Model file for the job. Use its own axes, mm. Coordinates: 2 decimals unless noted, no trailing zeros. Order: outer loops, then holes, each group sorted by start corner. A loop starts at its lowest first (then second) coordinate and runs counter-clockwise, first axis right, second up.
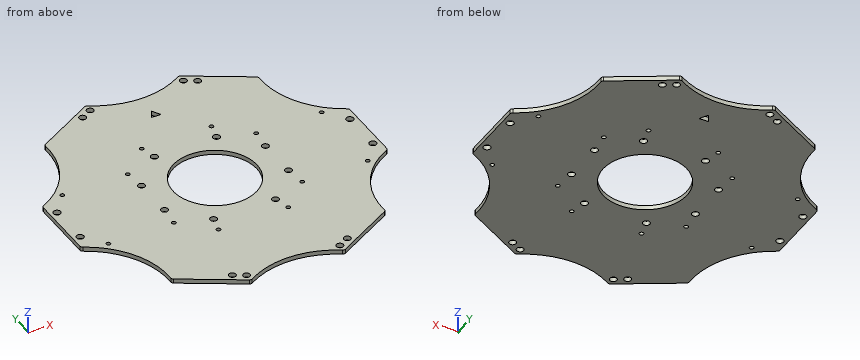
from build123d import *

# Parameters (mm, degrees)
SKETCH1_R           = 2.5
SKETCH1_R_2         = 2.6
SKETCH1_R_3         = 1.5
SKETCH1_R_4         = 30
BOSS_EXTRUDE1_DEPTH = 3.175
FILLET1_R           = 2


with BuildPart() as part:
    # Sketch1 → Boss-Extrude1 (new body)
    with BuildSketch(Plane.XY):
        with BuildLine():
            Line((-120, -25), (-120, 25))
            ThreePointArc((-120, 25), (-94.559451613, 48.820422151), (-86.650635095, 82.762794416))
            Line((-86.650635095, 82.762794416), (-43.349364905, 107.762794416))
            ThreePointArc((-43.349364905, 107.762794416), (-10, 97.640844302), (23.349364905, 107.762794416))
            Line((23.349364905, 107.762794416), (66.650635095, 82.762794416))
            ThreePointArc((66.650635095, 82.762794416), (74.559451613, 48.820422151), (100, 25))
            Line((100, 25), (100, -25))
            ThreePointArc((100, -25), (74.559451613, -48.820422151), (66.650635095, -82.762794416))
            Line((66.650635095, -82.762794416), (23.349364905, -107.762794416))
            ThreePointArc((23.349364905, -107.762794416), (-10, -97.640844302), (-43.349364905, -107.762794416))
            Line((-43.349364905, -107.762794416), (-86.650635095, -82.762794416))
            ThreePointArc((-86.650635095, -82.762794416), (-94.559451613, -48.820422151), (-120, -25))
        make_face()
        with Locations((12.227985364, -38.5)):
            Circle(SKETCH1_R, mode=Mode.SUBTRACT)
        with Locations((-54.455970728, 15)):
            Circle(SKETCH1_R, mode=Mode.SUBTRACT)
        with Locations((12.227985364, 38.5)):
            Circle(SKETCH1_R_2, mode=Mode.SUBTRACT)
        with Locations((-32.227985364, 38.5)):
            Circle(SKETCH1_R_2, mode=Mode.SUBTRACT)
        with Locations((-54.455970728, -15)):
            Circle(SKETCH1_R, mode=Mode.SUBTRACT)
        with Locations((-32.227985364, -38.5)):
            Circle(SKETCH1_R, mode=Mode.SUBTRACT)
        with Locations((95, 15)):
            Circle(SKETCH1_R_2, mode=Mode.SUBTRACT)
        with Locations((95, -15)):
            Circle(SKETCH1_R_2, mode=Mode.SUBTRACT)
        with Locations((-115, -15)):
            Circle(SKETCH1_R_2, mode=Mode.SUBTRACT)
        with Locations((-115, 15)):
            Circle(SKETCH1_R_2, mode=Mode.SUBTRACT)
        with Locations((31.241669751, -97.432667397)):
            Circle(SKETCH1_R, mode=Mode.SUBTRACT)
        with Locations((23.447441117, -101.932667397)):
            Circle(SKETCH1_R, mode=Mode.SUBTRACT)
        with Locations((-43.447441117, -101.932667397)):
            Circle(SKETCH1_R, mode=Mode.SUBTRACT)
        with Locations((-51.241669751, -97.432667397)):
            Circle(SKETCH1_R, mode=Mode.SUBTRACT)
        with Locations((-51.241669751, 97.432667397)):
            Circle(SKETCH1_R, mode=Mode.SUBTRACT)
        with Locations((-43.447441117, 101.932667397)):
            Circle(SKETCH1_R, mode=Mode.SUBTRACT)
        with Locations((23.447441117, 101.932667397)):
            Circle(SKETCH1_R, mode=Mode.SUBTRACT)
        with Locations((31.241669751, 97.432667397)):
            Circle(SKETCH1_R, mode=Mode.SUBTRACT)
        with Locations((34.455970728, -15)):
            Circle(SKETCH1_R, mode=Mode.SUBTRACT)
        with Locations((34.455970728, 15)):
            Circle(SKETCH1_R, mode=Mode.SUBTRACT)
        with Locations((-103, 30)):
            Circle(SKETCH1_R_3, mode=Mode.SUBTRACT)
        with Locations((-56, 30)):
            Circle(SKETCH1_R_3, mode=Mode.SUBTRACT)
        with Locations((-56, -30)):
            Circle(SKETCH1_R_3, mode=Mode.SUBTRACT)
        with Locations((-103, -30)):
            Circle(SKETCH1_R_3, mode=Mode.SUBTRACT)
        with Locations((36, 30)):
            Circle(SKETCH1_R_3, mode=Mode.SUBTRACT)
        with Locations((36, -30)):
            Circle(SKETCH1_R_3, mode=Mode.SUBTRACT)
        with Locations((83, 30)):
            Circle(SKETCH1_R_3, mode=Mode.SUBTRACT)
        with Locations((83, -30)):
            Circle(SKETCH1_R_3, mode=Mode.SUBTRACT)
        with Locations((-35, 50)):
            Circle(SKETCH1_R_3, mode=Mode.SUBTRACT)
        with Locations((15, 50)):
            Circle(SKETCH1_R_3, mode=Mode.SUBTRACT)
        with Locations((15, -50)):
            Circle(SKETCH1_R_3, mode=Mode.SUBTRACT)
        with Locations((-35, -50)):
            Circle(SKETCH1_R_3, mode=Mode.SUBTRACT)
        with Locations((-10, 0)):
            Circle(SKETCH1_R_4, mode=Mode.SUBTRACT)
        Polygon((-10, 82.640844302), (-13.464101615, 76.640844302), (-6.535898385, 76.640844302), align=None, mode=Mode.SUBTRACT)
    extrude(amount=BOSS_EXTRUDE1_DEPTH)

    # Fillet1
    fillet1_edges = [part.edges().sort_by_distance(p)[0] for p in [
        (-120, -25, 1.5875),
        (-120, 25, 1.5875),
        (-86.650635095, 82.762794416, 1.5875),
        (-43.349364905, 107.762794416, 1.5875),
        (23.349364905, 107.762794416, 1.5875),
        (66.650635095, 82.762794416, 1.5875),
        (100, 25, 1.5875),
        (100, -25, 1.5875),
        (66.650635095, -82.762794416, 1.5875),
        (23.349364905, -107.762794416, 1.5875),
        (-43.349364905, -107.762794416, 1.5875),
        (-86.650635095, -82.762794416, 1.5875),
    ]]
    fillet(fillet1_edges, radius=FILLET1_R)


solid = part.part
Q1. Probe line 1 (Y direction, x = 22, z = 1.6); line 2 (Y direction, x = 36, z = 0.9); line 3 (X direction, y = 30.5, z = 2.4). List the from-to ranges inside material, lowest first.
Established:
line 1: y = -106.89 to -103.97, -99.89 to 99.89, 103.97 to 106.89
line 2: y = -100.46 to -31.5, -28.5 to -16.97, -13.03 to 13.03, 16.97 to 28.5, 31.5 to 100.46
line 3: x = -110.95 to -104.41, -101.59 to -57.41, -54.59 to 34.59, 37.41 to 81.59, 84.41 to 90.95
Q2. Cut at A-A, the plane x = 95. List the corners of the cut face in (y, z) (3 decimals), plus the area to 3 significant figures.
Established:
outline: (-27.767, 0) - (-17.6, 0) - (-17.6, 3.175) - (-27.767, 3.175) - close; (-12.4, 0) - (12.4, 0) - (12.4, 3.175) - (-12.4, 3.175) - close; (17.6, 0) - (27.767, 0) - (27.767, 3.175) - (17.6, 3.175) - close
area: 143 mm2
Q3. Cut at B-B, the plane y = 38.5. List the corners of the cut face in (x, z) (3 decimals).
Established:
outline: (-102.088, 0) - (-34.828, 0) - (-34.828, 3.175) - (-102.088, 3.175) - close; (-29.628, 0) - (9.628, 0) - (9.628, 3.175) - (-29.628, 3.175) - close; (14.828, 0) - (82.088, 0) - (82.088, 3.175) - (14.828, 3.175) - close
Q4. Cut at C-C, the plane y = 15. List the corners of the cut face in (x, z) (3 decimals).
Established:
outline: (-120, 0) - (-117.6, 0) - (-117.6, 3.175) - (-120, 3.175) - close; (-112.4, 0) - (-56.956, 0) - (-56.956, 3.175) - (-112.4, 3.175) - close; (-51.956, 0) - (-35.981, 0) - (-35.981, 3.175) - (-51.956, 3.175) - close; (15.981, 0) - (31.956, 0) - (31.956, 3.175) - (15.981, 3.175) - close; (36.956, 0) - (92.4, 0) - (92.4, 3.175) - (36.956, 3.175) - close; (97.6, 0) - (100, 0) - (100, 3.175) - (97.6, 3.175) - close
Q5. Drop flat-ended pins along their axis: P1, Ø4.5, axis at x = -54.46, y = 15, coming from the +Z side; P2, Ø1.5, axis at x = -26, z = 1.5, coming from the -Y side. Give the stop position or say it passes through.
Established:
P1: passes through
P2: stops at y = -100.03
Q6. Cut at D-D, the plane z = 1. Count the separate pieces of the cut face and the enclosed holes in it, plus the area to 3 significant figures.
Established:
separate pieces: 1
enclosed holes: 34
area: 32,000 mm2
